```python
from build123d import *

# Parameters (mm, degrees)
SKETCH_R     = 2.75
PAD_DEPTH    = 3
SKETCH001_R  = 1.5
PAD001_DEPTH = 6
POCKET_DEPTH = 4


with BuildPart() as part:
    # Sketch → Pad (new body)
    with BuildSketch(Plane.XY):
        Circle(SKETCH_R)
    extrude(amount=PAD_DEPTH)

    # Sketch001 (on Face2 of Pad) → Pad001 (join)
    with BuildSketch(Plane(origin=(0, 0, 0), x_dir=(1, 0, 0), z_dir=(0, 0, -1))):
        Circle(SKETCH001_R)
    extrude(amount=PAD001_DEPTH)

    # Sketch002 (on DatumPlane) → Pocket (cut)
    with BuildSketch(Plane.XY.offset(3)):
        Polygon((0.721688, -1.25), (1.443376, 0), (0.721688, 1.25), (-0.721688, 1.25), (-1.443376, 0), (-0.721688, -1.25), align=None)
    extrude(amount=-POCKET_DEPTH, mode=Mode.SUBTRACT)


solid = part.part
```
Source: CAD feature listing. Evaluate the final solid. Frame: model axes, mm. A direction names the side the tool comes from. Give positions to 0.01 mm unless a question says otherwise; leave off trailing zeros. Loops run counter-clockwise (first coordinate to the right, second up) from the corner with the lowest first, then second, coordinate; pieces in that order, holes last. Notation, with made-up numbers: (-6, 8) - (44, 8) arc R10 cw to (44, 23) - close; hole circle Ø1 at (31, 65.25). An arc over 180 degrees is marked (long way). Use CSV: the item, a comma, the result in double quotes.
1) Cut plane B-B (x = 0). Output: boundary loops of the cut face in (y, z).
Worked out:
outline,"(-2.75, 0) - (-1.5, 0) - (-1.5, -6) - (1.5, -6) - (1.5, 0) - (2.75, 0) - (2.75, 3) - (1.25, 3) - (1.25, -1) - (-1.25, -1) - (-1.25, 3) - (-2.75, 3) - close"
2) Pin query (flat end, axial travel): P1, Ø1.5, axis at x = -1, z = -4.5, coming from the +Y side. Return the tip coordinate at first contact, or that it passes through.
Worked out:
P1,"stops at y = 1.48"
3) Cut plane A-A (z = -0.25). Output: boundary loops of the cut face in (x, y), and give its area (3 significant figures).
Worked out:
outline,"circle Ø3 at (0, 0); hole (-1.44, 0) - (-0.72, -1.25) - (0.72, -1.25) - (1.44, 0) - (0.72, 1.25) - (-0.72, 1.25) - close"
area,"1.66 mm^2"
4) Set-up query: faces 4 (the cylindrical face through (-1.5, -0.07, -2.96)), 5 (the flat face through (-1.3, -0.6, 3)), 6 (the flat face through (-1.088, -0.616, 1.028)). Return all of +Z, -Z, +X, -X, +Y, -Y with unobstructed straight access to the full face (end or side cutting, diameter ignored); none if empty.
Worked out:
face 4,"-Z"
face 5,"+Z, +X, -X, +Y, -Y"
face 6,"+Z"
5) Cut plane C-C (y = 0.7). Output: boundary loops of the cut face in (x, z), and give its area (3 significant figures).
Worked out:
outline,"(-2.66, 0) - (-1.33, 0) - (-1.33, -6) - (1.33, -6) - (1.33, 0) - (2.66, 0) - (2.66, 3) - (1.04, 3) - (1.04, -1) - (-1.04, -1) - (-1.04, 3) - (-2.66, 3) - close"
area,"23.6 mm^2"
6) Cut plane D-D (z = -5.25). Output: boundary loops of the cut face in (x, y), and give its area (3 significant figures).
Worked out:
outline,"circle Ø3 at (0, 0)"
area,"7.07 mm^2"
7) Line query: line 1 (X direction, y = 0.4, z = -3.5); line 2 (Z direction, x = -2.45, y = -1.1); line 3 (Y direction, x = 0.85, z = 2.5). Output: solid intervals per line, ascending.
Worked out:
line 1,"x = -1.45 to 1.45"
line 2,"z = 0 to 3"
line 3,"y = -2.62 to -1.03, 1.03 to 2.62"
8) Mould query, pull axis X, two halves, no side actions, for faces 1 (the flat face through (1.2, -1.2, 0)), 2 (the cylindrical face through (-0.596, -2.685, 1.479)), 3 (the flat face through (1.088, 0.616, 1.028)). Classes: +X half, -X half, draft (parallel to the pull), parting line (faces both ways), or undercut.
Worked out:
face 1,"draft"
face 2,"parting line"
face 3,"undercut"
